Source: CAD feature listing. Evaluate the final solid. Frame: model axes, mm. Face numbers are marked on the shaded views. A direction names the side the tool comes from. Coordinates: 2 decimals unless noted, no trailing zeros. Loops run counter-clockwise (first coordinate to the right, second up) from the corner with the lowest first, then second, coordinate; pieces in that order, holes last.
Item 1: Line query: probe 1 along Y at (x, z) = (4.5, 0); probe 2 along Z at (x, y) = (0, 11.5); probe 3 along Y at (x, z) = (4, -2.25). Output: solid intervals per line, ascending.
Item 2: Pin query (flat end, axial travel): pin 1 Ø8 at (x, y) = (5.5, 27.5) entering from -Z; pin 2 Ø4 at (y, z) = (10, 0) entering from -X; pin 3 Ø3 at (x, y) = (-6, 28.5) entering from -Z; pin 4 Ø5 at (x, y) = (0.5, 35) entering from +Z. Return the tip coordinate at first contact, or that it passes through.
Item 3: Section query B-B, the plane y = 36.5. Return the cut outline in (x, z), then the cut area to 3 significant figures.
Item 4: Section query A-A, the plane y = 10. Return the cut outline in (x, z), then the cut area to 3 significant figures.
Item 5: Reachability of the marked faces 1, 2, 3, 4 and 5 from +Z, -Z, +X, -X, +Y, -Y: full face, straight path, thin tool, end or side. Return the list, or none.
Item 6: Pull-direction query (Z, two-part tool) for the marked faces 6, 7 and 8; classes: +Z half, -Z half, draft (parallel to the pull), parting line (faces both ways), or undercut.
```python
from build123d import *

# Parameters (mm, degrees)
F0_R            = 8
F1_DEPTH        = 20
F2_R            = 5
F3_DEPTH        = 20
F5_DEPTH        = 16
F5_COPIES_COUNT = 3
F6_SIZE         = 0.49999
F7_R            = 0.5
F9_D            = 5
F9_DEPTH        = 14
F9_TIP          = 1.5021515476
F10_R           = 2.1
F11_DEPTH       = 8.25
F12_SIZE        = 3


# Not quite as in the source:
# - a fillet or chamfer is up to 0.001 mm smaller than in the source, because OpenCascade refuses the exact size
# - a pattern or mirror of a feature is missing from the dataset's text; its kind, count and spacing are read off the source's solid


with BuildPart() as f1:
    # F0 (on Front) → F1 (new body)
    with BuildSketch(Plane.XZ):
        Circle(F0_R)
    extrude(amount=-F1_DEPTH)

    # F2 (on face) → F3 (join)
    with BuildSketch(Plane(origin=(0, 20, 0), x_dir=(-1, 0, 0), z_dir=(0, 1, 0))):
        Circle(F2_R)
    extrude(amount=F3_DEPTH)

    # F4 (on face) → F5 (cut)
    with BuildSketch(Plane(origin=(0, 40, 0), x_dir=(-1, 0, 0), z_dir=(0, 1, 0))):
        with BuildLine():
            ThreePointArc((2.1794494718, 4.5), (0, 5), (-2.1794494718, 4.5))
            Line((-2.1794494718, 4.5), (2.1794494718, 4.5))
        make_face()
    f5 = extrude(amount=-F5_DEPTH, mode=Mode.SUBTRACT)

    # F5_copies: F5 ×3 about axis
    f5_copies_axis = Axis((0, 0, 0), (0, 1, 0))
    for i in range(1, F5_COPIES_COUNT):
        add(f5.rotate(f5_copies_axis, i * 360 / F5_COPIES_COUNT), mode=Mode.SUBTRACT)

    # F6 (size 0.5 in the source; OpenCascade refuses exactly that, so slightly less here)
    f6_edges = [f1.edges().sort_by_distance(p)[0] for p in [
        (4.330127, 40, 2.5),
        (-4.996709, 40, -0.18139),
        (0, 40, -5),
        (-4.236582, 40, 2.655443),
    ]]
    chamfer(f6_edges, length=F6_SIZE)

    # F7
    f7_edges = [f1.edges().sort_by_distance(p)[0] for p in [
        (-8, 20, 0),
        (5, 20, 0),
    ]]
    fillet(f7_edges, radius=F7_R)

    # F9
    with Locations(Plane.XZ):
        with Locations((0, 0)):
            Hole(F9_D / 2, depth=F9_DEPTH)
            with Locations((0, 0, -(F9_DEPTH + F9_TIP / 2))):  # 118° drill point
                Cone(0, F9_D / 2, F9_TIP, mode=Mode.SUBTRACT)

    # F10 (on Right) → F11 (cut, symmetric)
    with BuildSketch(Plane.YZ):
        with Locations((10, 0)):
            Circle(F10_R)
    extrude(amount=F11_DEPTH, both=True, mode=Mode.SUBTRACT)

    # F12
    f12_edges = [f1.edges().sort_by_distance(p)[0] for p in [
        (-8, 0, 0),
    ]]
    chamfer(f12_edges, length=F12_SIZE)


solid = f1.part
```
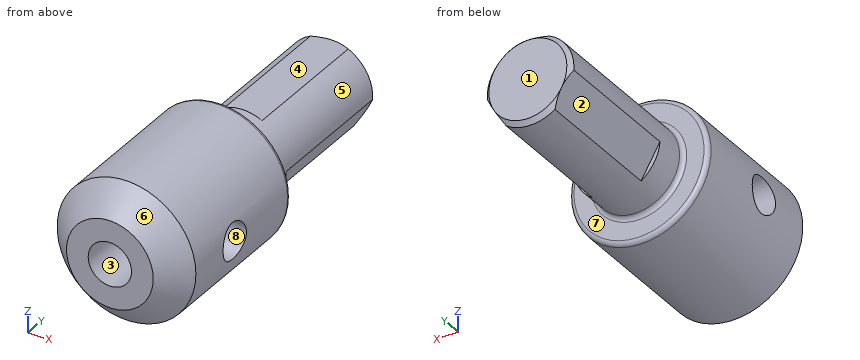
Verdict:
1. probe 1: y = 0 to 7.9, 12.1 to 40
1. probe 2: z = -8 to -2.5, 2.5 to 8
1. probe 3: y = 0 to 24
2. pin 1: stops at z = -4.77
2. pin 2: passes through
2. pin 3: stops at z = -1.21
2. pin 4: stops at z = 4.5
3. outline: (-4.99, -0.36) - (-2.81, -4.14) arc R5 ccw to (2.81, -4.14) - (4.99, -0.36) arc R5 ccw to (2.18, 4.5) - (-2.18, 4.5) arc R5 ccw to start
3. area: 74.1 mm2
4. outline: (-7.72, -2.1) arc R8 ccw to (7.72, -2.1) - (1.36, -2.1) arc R2.5 cw to (-1.36, -2.1) - close; (-7.72, 2.1) - (-1.36, 2.1) arc R2.5 cw to (1.36, 2.1) - (7.72, 2.1) arc R8 ccw to start
4. area: 133 mm2
5. face 1: +Z, -Z, +X, -X, +Y
5. face 2: -Z, -X, +Y
5. face 3: -Y
5. face 4: +Z, +X, -X, +Y
5. face 5: +Y
6. face 6: parting line
6. face 7: draft
6. face 8: undercut
